Autodesk Inventor part; units mm, degrees
ref_plane "YZ Plane" through (0, 0, 0) normal (1, 0, 0) x (0, 1, 0)
ref_plane "XZ Plane" through (0, 0, 0) normal (0, 1, 0) x (-1, 0, 0)
ref_plane "XY Plane" through (0, 0, 0) normal (0, 0, 1) x (1, 0, 0)
ref_plane "Arbeitsebene1" through (0, 0, 0) normal (0, 0, 1) x (1, 0, 0)
sketch "Skizze1" plane through (0, 0, 0) normal (0, 0, 1) x (1, 0, 0)
  line L0 (-0.2844, 28.5315) -> (-56.8529, 85.1)
  circle A0 centre (-11.3693, 45.2732) radius 1.49
  circle A1 centre (-41.3693, 75.2732) radius 1.4
  line L1 (-47.0261, 75.2732) -> (-41.3693, 80.9301)
  line L2 (-41.3693, 80.9301) -> (-5.7124, 45.2732)
  line L3 (-5.7124, 45.2732) -> (-11.3693, 39.6164)
  line L4 (-11.3693, 39.6164) -> (-47.0261, 75.2732)
  line L5 (-51.5685, 65.6735) -> (5, 9.105)
  line L6 (-47.0261, 75.2732) -> (-54.0972, 68.2022)
  line L7 (-54.0972, 68.2022) -> (-18.4403, 32.5453)
  line L8 (-18.4403, 32.5453) -> (-11.3693, 39.6164)
  line L9 (-11.3693, 39.6164) -> (-47.0261, 75.2732)
  point P0 (0, 0)
  dimension "d0" = 4
  dimension "d1" = 4
  dimension "d2" = 4
  dimension "d3" = 4
extrude "Extrusion1" add sketch "Skizze1" along normal blind 10
properties part number "NematostellaImager_mirrormount"
Source: CAD feature listing. Evaluate the final solid. Frame: model axes, mm. Give positions to 0.01 mm unless a question says otherwise; leave off trailing zeros. Write each loop counter-clockwise with the first axis right and the second up, starting at its lowest first coordinate (ties: lowest second). Pieces come first, ordered by that corner, then holes. Notation, with made-up numbers: M 7.25,30.5 L 61.25,30.5 A28 cw 61.25,48.5 Z; hole C -26.75,27.25 d9. An arc over 180 degrees is marked long. Return JSON: item names as keys, results as strings. Group by question number.
1) Cut plane A-A, the plane z = 2.75. Output: boundary loops of the cut face in (x, y), then the cut area to 3 significant figures.
2) Ray query, L1, parallel to X at y = 75.5, z = 8.25; L2, parallel to Y at x = -41, z = 3.75 (3 decimals); L3, parallel to Y at x = -47.5, z = 5.25 (3 decimals). Return the intervals inside material, ascending.
3) Cut plane C-C, the plane x = -24.5. Output: boundary loops of the cut face in (y, z) (3 decimals).
4) Cut plane B-B, the plane y = 46. Output: boundary loops of the cut face in (x, z) (3 decimals).
5) Draft query along X for faces 1 (the face through (-36.518, 50.623, 4.93)), 2 (the face through (-41.552, 73.885, 4.93)), 3 (the face through (-30, 57, 0)). Return one class per face: released by +X, released by -X, zero draft, split by the parting line, or undercut.
6) Cut plane D-D, the plane x = -49. Output: boundary loops of the cut face in (y, z) (3 decimals).
7) First-contact query: pin 1 Ø4 at (x, z) = (-31, 6.5) entering from +Y; pin 2 Ø1 at (y, z) = (75, 4) entering from +X; pin 3 Ø2 at (y, z) = (53.5, 3) entering from -X (3 decimals). Flat tips, straight axial feed; report the tip coordinate or a pass-through.
Data:
{
 "1": {"outline": "M -54.1,68.2 L -18.44,32.55 L -11.37,39.62 L -5.71,45.27 L -41.37,80.93 L -47.03,75.27 Z; hole C -41.37,75.27 d2.8; hole C -11.37,45.27 d2.98", "area": "895 mm²"},
 "2": {"L1": "x = -46.8 to -42.75, -39.99 to -35.94", "L2": "y = 55.105 to 73.923, 76.624 to 80.561", "L3": "y = 61.605 to 74.799"},
 "3": {"outline": "M 38.605,0 L 64.061,0 L 64.061,10 L 38.605,10 Z"},
 "4": {"outline": "M -31.895,0 L -12.67,0 L -12.67,10 L -31.895,10 Z; M -10.069,0 L -6.439,0 L -6.439,10 L -10.069,10 Z"},
 "5": {"face 1": "released by -X", "face 2": "undercut", "face 3": "zero draft"},
 "6": {"outline": "M 63.105,0 L 73.299,0 L 73.299,10 L 63.105,10 Z"},
 "7": {"pin 1": "stops at y = 72.56", "pin 2": "stops at x = -34.94", "pin 3": "stops at x = -40.395"}
}
